```python
from build123d import *

# Parameters (mm, degrees)
BOSS_EXTRUDE1_DEPTH = 3
SKETCH2_W           = 3
SKETCH2_H           = 4.17
BOSS_EXTRUDE2_DEPTH = 3
CUT_EXTRUDE2_DEPTH  = 3
CHAMFER1_SIZE       = 4


with BuildPart() as part:
    # Sketch1 → Boss-Extrude1 (new body)
    with BuildSketch(Plane.XY):
        Polygon((0, 14.5), (0, -0.717472322), (17.74276268, -24.90826339), (25, -19.585434587), align=None)
    extrude(amount=-BOSS_EXTRUDE1_DEPTH)

    # Sketch2 → Boss-Extrude2 (add)
    with BuildSketch(Plane.XY):
        with Locations((-1.5, 6.891263839)):
            Rectangle(SKETCH2_W, SKETCH2_H)
    extrude(amount=-BOSS_EXTRUDE2_DEPTH)

    # Sketch3 → Cut-Extrude2 (cut)
    with BuildSketch(Plane(origin=(0, 0, -3), x_dir=(-1, 0, 0), z_dir=(0, 0, -1))):
        Polygon((-13.427123713, -3.806773881), (-17.200564762, -8.951549002), (-15.495347423, -14.704133971), (-11.12785759, -11.563394363), align=None)
    extrude(amount=-CUT_EXTRUDE2_DEPTH, mode=Mode.SUBTRACT)

    # Chamfer1
    chamfer1_edges = [part.edges().sort_by_distance(p)[0] for p in [
        (25, -19.585434587, -1.5),
    ]]
    chamfer(chamfer1_edges, length=CHAMFER1_SIZE)


solid = part.part
```
For this review, take the finished solid that the model builds, in its own axes (mm). A direction names the side the tool comes from. Coordinates: 2 decimals unless noted, no trailing zeros. Order: outer loops, then holes, each group sorted by start corner. A loop starts at its lowest first (then second) coordinate and runs counter-clockwise, first axis right, second up. Notation, with made-up numbers: (-13, 3.5) -> (6, 3.5) arc R22 ccw to (6, 39.5) -> close; hole circle Ø4 at (50.25, 24). An arc over 180 degrees is marked (long way). Use CSV: the item, a comma, the result in double quotes. Start each with the question number.
Item 1: We need section A-A, the plane z = -1.9. Give the boundary of the cut face in (x, y).
Item 2: We need section B-B, the plane y = 11. Give the boundary of the cut face in (x, z), then the cut area to 3 significant figures.
Item 3: Draft analysis for pull direction X (two halves, no side actions). For faces 1 (the face through (16.36, -11.79, -1.52)), 2 (the face through (0, 12, -1)), 3 (the face through (19.73, -23.45, -1.48)), state which applies: pulls with the +X half, pulls with the -X half, needs draft (parallel to the pull), parting line crosses it, or undercut.
Item 4: We need section C-C, the plane x = 20.5. Give the boundary of the cut face in (y, z), then the cut area to 3 significant figures.
Item 5: Insertion check: pin 1 (1.5 mm diameter, centred on y = 0, z = -2, fed in from +X). The pin has a flat end and moves straight along its axis. Give the tip position at first contact, or say it passes through.
Item 6: For faces 4 (the face through (-2, 8.976, -1)), 5 (the face through (13.342, -13.156, -1.521)), 6 (the face through (-2, 4.806, -1)), list the 3-axis set-ups (+Z, -Z, +X, -X, +Y, -Y) from which the entire face can be reached by the end or side of a thin tool; tool diameter is ignored.
Item 7: Wall thickness on probe 1 along Y at (x, z) = (-1.25, -1.4); probe 2 along X at (y, z) = (-14.5, -1.35); probe 3 along Y at (x, z) = (17.5, -2): over which ranges is each line inside the solid? List them lowest first.
Derived:
1,outline,"(-3, 4.81) -> (0, 4.81) -> (0, -0.72) -> (17.74, -24.91) -> (21.77, -21.95) -> (22.63, -16.36) -> (17.2, -8.95) -> (15.5, -14.7) -> (11.13, -11.56) -> (13.43, -3.81) -> (0, 14.5) -> (0, 8.98) -> (-3, 8.98) -> close"
2,outline,"(0, -3) -> (2.57, -3) -> (2.57, 0) -> (0, 0) -> close"
2,area,"7.70 mm^2"
3,face 1,"undercut"
3,face 2,"pulls with the -X half"
3,face 3,"pulls with the +X half"
4,outline,"(-22.89, -3) -> (-13.45, -3) -> (-13.45, 0) -> (-22.89, 0) -> close"
4,area,"28.3 mm^2"
5,pin 1,"stops at x = 11.19"
6,face 4,"+Z, -Z, -X, +Y"
6,face 5,"+Z, -Z"
6,face 6,"+Z, -Z, -X, -Y"
7,probe 1,"y = 4.81 to 8.98"
7,probe 2,"x = 10.11 to 15.21, 15.56 to 21.27"
7,probe 3,"y = -24.58 to -9.36"
